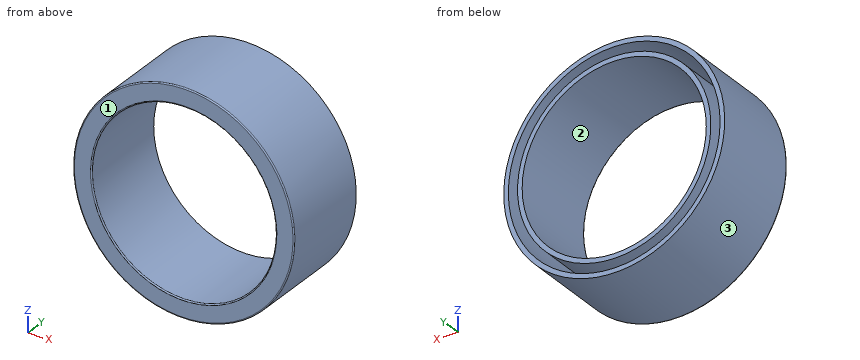
from build123d import *

# Parameters (mm, degrees)
SKETCH1_R           = 24
SKETCH1_R_2         = 20
BOSS_EXTRUDE1_DEPTH = 20
SHELL4_T            = -1
FILLET1_R           = 0.25
FILLET2_R           = 0.25


with BuildPart() as part:
    # Sketch1 → Boss-Extrude1 (new body)
    with BuildSketch(Plane(origin=(0, 0, 0), x_dir=(1, 0, 0), z_dir=(0, 1, 0))):
        with Locations(Location((0, 0, 0), (0, 0, 270))):
            Circle(SKETCH1_R)
        with Locations(Location((0, 0, 0), (0, 0, 270))):
            Circle(SKETCH1_R_2, mode=Mode.SUBTRACT)
    extrude(amount=-BOSS_EXTRUDE1_DEPTH)

    # Shell4
    shell4_openings = [part.faces().sort_by_distance(p)[0] for p in [
        (0, 0, -23.32117749),
    ]]
    offset(amount=SHELL4_T, openings=shell4_openings, kind=Kind.INTERSECTION)

    # Fillet1
    fillet1_edges = [part.edges().sort_by_distance(p)[0] for p in [
        (0, -20, -20),
    ]]
    fillet(fillet1_edges, radius=FILLET1_R)

    # Fillet2
    fillet2_edges = [part.edges().sort_by_distance(p)[0] for p in [
        (0, -20, -24),
    ]]
    fillet(fillet2_edges, radius=FILLET2_R)


solid = part.part
Could you check a few things on this model? Use its own coordinates, in mm. Face numbers are marked on the shaded views. Give positions to 0.01 mm unless a question says otherwise; leave off trailing zeros. Loops run counter-clockwise (first coordinate to the right, second up) from the corner with the lowest first, then second, coordinate; pieces in that order, holes last. Notation, with made-up numbers: M 57,63.5 L 65,63.5 A37 ccw 65,101.5 Z; hole C 60.5,-22 d11. An arc over 180 degrees is marked long. Answer as a JSON object with one key per item and string values.
Q1. If I drill on probe 1 along X at (y, z) = (-15.5, 0); probe 2 along Z at (x, y) = (-0.5, -18.5); probe 3 along X at (y, z) = (-5, -7) (3 decimals), over which ranges is the centre line in solid material (lowest first)? Write a range as [from, to].
Values found:
{"probe 1": "x = [-24, -23], [-21, -20], [20, 21], [23, 24]", "probe 2": "z = [-23.99, -22.99], [-20.99, -19.99], [19.99, 20.99], [22.99, 23.99]", "probe 3": "x = [-22.956, -21.909], [-19.799, -18.735], [18.735, 19.799], [21.909, 22.956]"}
Q2. Suppose I cut it at C-C, the plane x = 0. List the corners of the cut face in (y, z) for me, plus the area to 3 significant figures.
Values found:
{"outline": "M -20,-23.75 A0.25 ccw -19.75,-24 L 0,-24 L 0,-23 L -19,-23 L -19,-21 L 0,-21 L 0,-20 L -19.75,-20 A0.25 ccw -20,-20.25 Z; M -20,20.25 A0.25 ccw -19.75,20 L 0,20 L 0,21 L -19,21 L -19,23 L 0,23 L 0,24 L -19.75,24 A0.25 ccw -20,23.75 Z", "area": "83.9 mm²"}
Q3. Suppose I cut it at A-A, the plane z = 0. List the corners of the cut face in (x, y) for me.
Values found:
{"outline": "M -24,-19.75 A0.25 ccw -23.75,-20 L -20.25,-20 A0.25 ccw -20,-19.75 L -20,0 L -21,0 L -21,-19 L -23,-19 L -23,0 L -24,0 Z; M 20,-19.75 A0.25 ccw 20.25,-20 L 23.75,-20 A0.25 ccw 24,-19.75 L 24,0 L 23,0 L 23,-19 L 21,-19 L 21,0 L 20,0 Z"}
Q4. If we mould it in two halves opening along Z, with no side actions, what happens to the marked faces 1, 2 and 3? For each: pulls with the +Z half, pulls with the -Z half, needs draft (parallel to the pull), parting line crosses it, or undercut.
Values found:
{"face 1": "needs draft", "face 2": "undercut", "face 3": "parting line crosses it"}
Q5. For P1, Ø4, axis at y = -17.5, z = -11.5, coming from the +X side; P2, Ø10, axis at y = -11, z = -12, coming from the -X side; P3, Ø4, axis at x = -14.5, y = -14, coming from the +Z side; P4, Ø23, axis at x = 0, z = -2, coming from the +Y side, each with a flat end and sliding along its axis, tell me the tip position at first contact or that it passes through.
Values found:
{"P1": "stops at x = 22.04", "P2": "stops at x = -22.96", "P3": "stops at z = 20.49", "P4": "passes through"}
Q6. Suppose I cut it at B-B, the plane y = -4.5. List the corners of the cut face in (x, z) for me.
Values found:
{"outline": "C 0,0 d48; C 0,0 d42; hole C 0,0 d46; hole C 0,0 d40"}
